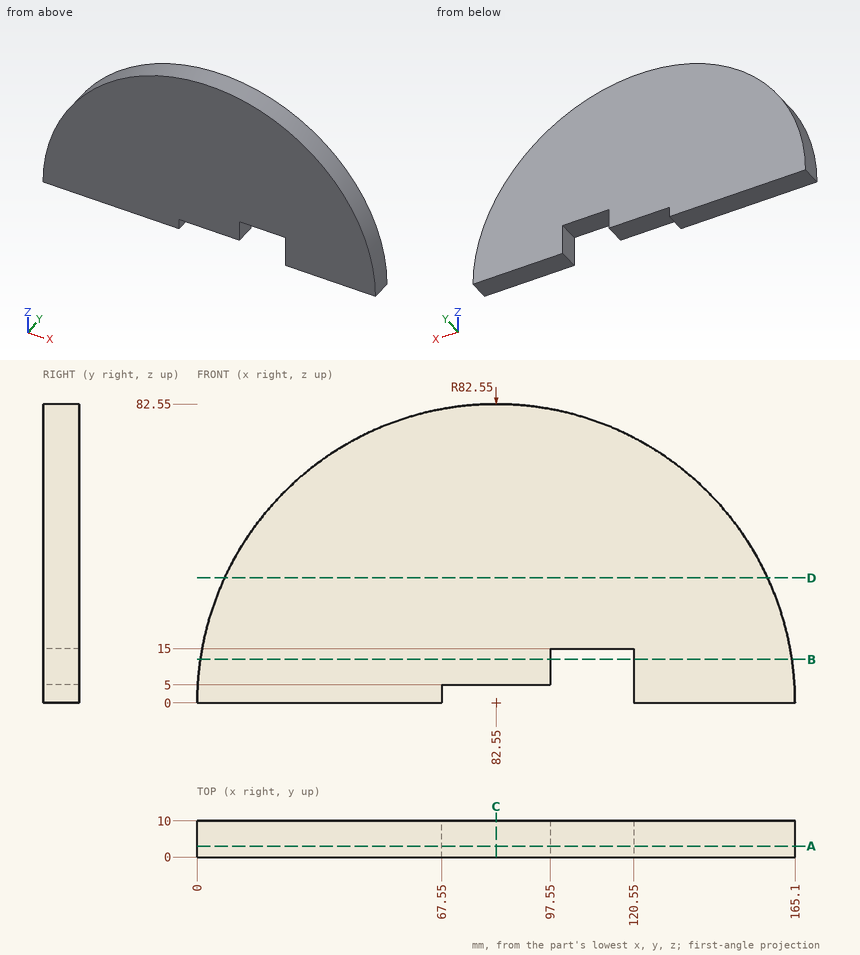
Geometry check sheet. Reference: drawing and pictorial views, mm from the part's lowest x, y, z. Give positions to 0.01 mm unless a question says otherwise; leave off trailing zeros. Write each loop counter-clockwise with the first axis right and the second up, starting at its lowest first coordinate (ties: lowest second). Pieces come first, ordered by that corner, then holes. Notation, with made-up numbers: M -5.5,13.5 L 29.5,13.5 A19 ccw 29.5,38.5 Z; hole C -3,36 d5. An arc over 180 degrees is marked long. Answer as CSV lines item,"result". Start each with the question number.
Q1. Material ranges on L1, parallel to Z at x = 81, y = 9; L2, parallel to X at y = 6.75, z = 11.5; L3, parallel to X at y = 6.5, z = 10.5, recorded low to high.
Q2. Section check B-B, the plane z = 12. Record the cut outline in (x, y).
Q3. Go/stop test with flat-tipped pins: pin 1 (2.5 mm diameter, centred on y = 6.5, z = 2.5, fed in from +X); pin 2 (3 mm diameter, centred on y = 4, z = 12, fed in from +X); pin 3 (6 mm diameter, centred on y = 6, z = 22.5, fed in from +X); pin 4 (8 mm diameter, centred on x = 75.5, z = 69.5, fed in from -Y). Record where each tip stops, or that it passes through.
Q4. Section check A-A, the plane y = 3. Record the cut outline in (x, z), then the cut area to 3 significant figures.
Q5. Section check D-D, the plane z = 34.5. Record the cut outline in (x, y), then the cut area to 3 significant figures.
Q6. Section check C-C, the plane x = 82.55. Record the cut outline in (y, z), then the cut area to 4 significant figures.
Geometry says:
1,L1,"5 to 82.54"
1,L2,"0.8 to 97.55, 120.55 to 164.3"
1,L3,"0.67 to 97.55, 120.55 to 164.43"
2,outline,"M 0.88,0 L 97.55,0 L 97.55,10 L 0.88,10 Z; M 120.55,0 L 164.22,0 L 164.22,10 L 120.55,10 Z"
3,pin 1,"x = 165.09"
3,pin 2,"x = 164.43"
3,pin 3,"x = 162.76"
3,pin 4,"y = 0"
4,outline,"M 0,0 L 67.55,0 L 67.55,5 L 97.55,5 L 97.55,15 L 120.55,15 L 120.55,0 L 165.1,0 A82.55 ccw Z"
4,area,"10,200 mm^2"
5,outline,"M 7.55,0 L 157.55,0 L 157.55,10 L 7.55,10 Z"
5,area,"1,500 mm^2"
6,outline,"M 0,5 L 10,5 L 10,82.55 L 0,82.55 Z"
6,area,"775.5 mm^2"
